```python
from build123d import *

# Parameters (mm, degrees)
SKETCH_1_R      = 1.6
EXTRUDE_1_DEPTH = 3
SKETCH_2_R      = 1.8
EXTRUDE_2_DEPTH = 3
FILLET_1_R      = 2


with BuildPart() as part:
    # 草图1 → 凸台-拉伸1 (new body)
    with BuildSketch(Plane(origin=(0, 0, 0), x_dir=(0, 0, -1), z_dir=(1, 0, 0))):
        with BuildLine():
            Line((-20, 0), (20, 0))
            Line((20, 0), (20, 27))
            ThreePointArc((20, 27), (0, 47), (-20, 27))
            Line((-20, 27), (-20, 0))
        make_face()
        with Locations((-7.75, 40.423393759)):
            Circle(SKETCH_1_R, mode=Mode.SUBTRACT)
        with Locations((7.75, 40.423393759)):
            Circle(SKETCH_1_R, mode=Mode.SUBTRACT)
        with Locations((15.5, 27)):
            Circle(SKETCH_1_R, mode=Mode.SUBTRACT)
        with Locations((7.75, 13.576606241)):
            Circle(SKETCH_1_R, mode=Mode.SUBTRACT)
        with Locations((-7.75, 13.576606241)):
            Circle(SKETCH_1_R, mode=Mode.SUBTRACT)
        with Locations((-15.5, 27)):
            Circle(SKETCH_1_R, mode=Mode.SUBTRACT)
        with BuildLine():
            Line((6.5, 32.5), (6.5, 18.5))
            ThreePointArc((6.5, 18.5), (0, 12), (-6.5, 18.5))
            Line((-6.5, 18.5), (-6.5, 32.5))
            ThreePointArc((-6.5, 32.5), (0, 39), (6.5, 32.5))
        make_face(mode=Mode.SUBTRACT)
    extrude(amount=EXTRUDE_1_DEPTH)

    # 草图2 → 凸台-拉伸2 (add)
    with BuildSketch(Plane.XZ):
        with BuildLine():
            Line((0, 20), (41, 20))
            ThreePointArc((41, 20), (42.414213562, 19.414213562), (43, 18))
            Line((43, 18), (43, -18))
            ThreePointArc((43, -18), (42.414213562, -19.414213562), (41, -20))
            Line((41, -20), (0, -20))
            Line((0, -20), (0, 20))
        make_face()
        with Locations(Location((11, 15, 0), (0, 0, 270))):
            Circle(SKETCH_2_R, mode=Mode.SUBTRACT)
        with Locations(Location((35, 15, 0), (0, 0, 270))):
            Circle(SKETCH_2_R, mode=Mode.SUBTRACT)
        with Locations(Location((11, -15, 0), (0, 0, 270))):
            Circle(SKETCH_2_R, mode=Mode.SUBTRACT)
        with Locations(Location((35, -15, 0), (0, 0, 270))):
            Circle(SKETCH_2_R, mode=Mode.SUBTRACT)
    extrude(amount=-EXTRUDE_2_DEPTH)

    # 圆角1
    fillet_1_edges = [part.edges().sort_by_distance(p)[0] for p in [
        (0, 0, 0),
        (3, 3, 0),
    ]]
    fillet(fillet_1_edges, radius=FILLET_1_R)


solid = part.part
```
For this review, take the finished solid that the model builds, in its own axes (mm). A direction names the side the tool comes from. Coordinates: 2 decimals unless noted, no trailing zeros. Write each loop counter-clockwise with the first axis right and the second up, starting at its lowest first coordinate (ties: lowest second). Pieces come first, ordered by that corner, then holes. Notation, with made-up numbers: (-31.75, 30) -> (22.25, 30) arc R18 cw to (22.25, 45) -> close; hole circle Ø6 at (41, 23.25). An arc over 180 degrees is marked (long way). Put each result on its own line as item: value.
Q1. Take a section at B-B, the plane z = -15. State the section outline as (x, y) points.
From the geometry:
outline: (0, 2) arc R2 ccw to (2, 0) -> (9.2, 0) -> (9.2, 3) -> (5, 3) arc R2 cw to (3, 5) -> (3, 25.48) -> (0, 25.48) -> close; (0, 28.52) -> (3, 28.52) -> (3, 40.23) -> (0, 40.23) -> close; (12.8, 0) -> (33.2, 0) -> (33.2, 3) -> (12.8, 3) -> close; (36.8, 0) -> (43, 0) -> (43, 3) -> (36.8, 3) -> close
Q2. Wall thickness on L1, parallel to X at y = 2.25, z = -15; L2, parallel to Y at x = 11.5, z = -4: over which ranges is each line inside the solid? List them lowest first.
From the geometry:
L1: x = 0 to 9.2, 12.8 to 33.2, 36.8 to 43
L2: y = 0 to 3
Q3. Tool access review of faces 4 (the cylindrical face through (9.243, 1.479, 15.39)), 5 (the flat face through (24, 3, 0)), 6 (the cylindrical face through (1, 39, 0)): name each direction out of +Z, -Z, +X, -X, +Y, -Y from which nothing blocks a thin tool from reaching the whole face with its end or side.
From the geometry:
face 4: +Y, -Y
face 5: +Z, -Z, +X, +Y
face 6: +X, -X
Q4. The part is to be moulded in two halves that separate along Z. For faces 1 (the cylindrical face through (3.6, 3.57, 0.28)), 2 (the flat face through (1, 26, -6.5)), 3 (the cylindrical face through (1, 47, 0)), say which applies: +Z half, -Z half, draft (parallel to the pull), parting line (faces both ways), or undercut.
From the geometry:
face 1: draft
face 2: undercut
face 3: parting line
Q5. Clearance check with a flat-ended pin moving along its axis: pin 1 Ø6 at (x, z) = (35, 8.5) entering from +Y. State where the tip first meets the part, or that it passes through.
From the geometry:
pin 1: stops at y = 3
Q6. Take a section at C-C, the plane y = 37. State the section outline as (x, z) points, then the cut area to 3 significant figures.
From the geometry:
outline: (0, -17.32) -> (3, -17.32) -> (3, -4.69) -> (0, -4.69) -> close; (0, 4.69) -> (3, 4.69) -> (3, 17.32) -> (0, 17.32) -> close
area: 75.8 mm2
Q7. Take a section at A-A, the plane x = 35. State the section outline as (y, z) points.
From the geometry:
outline: (0, -20) -> (3, -20) -> (3, -16.8) -> (0, -16.8) -> close; (0, -13.2) -> (3, -13.2) -> (3, 13.2) -> (0, 13.2) -> close; (0, 16.8) -> (3, 16.8) -> (3, 20) -> (0, 20) -> close
Q8. Take a section at D-D, the plane z = 7.75. State the section outline as (x, y) points.
From the geometry:
outline: (0, 2) arc R2 ccw to (2, 0) -> (43, 0) -> (43, 3) -> (5, 3) arc R2 cw to (3, 5) -> (3, 11.98) -> (0, 11.98) -> close; (0, 15.18) -> (3, 15.18) -> (3, 38.82) -> (0, 38.82) -> close; (0, 42.02) -> (3, 42.02) -> (3, 45.44) -> (0, 45.44) -> close
